For this review, take the finished solid that the model builds, in its own axes (mm). Round coordinates to 2 decimals unless told otherwise and drop trailing zeros. Loops run counter-clockwise (first coordinate to the right, second up) from the corner with the lowest first, then second, coordinate; pieces in that order, holes last. Notation, with made-up numbers: (42.25, 89) -> (47.25, 89) arc R8 ccw to (47.25, 95) -> close; hole circle Ø8 at (9, -16.5). An arc over 180 degrees is marked (long way). Use one line per item in the form item = value. Start each with the question number.
from build123d import *

# Parameters (mm, degrees)
F1_DEPTH = 20
F2_R     = 5
F4_DEPTH = 18


with BuildPart() as f1:
    # F0 (on Top) → F1 (new body)
    with BuildSketch(Plane.XY):
        Polygon((3.5849593993, 10.2129992476), (-4.6867319226, 9.7566301257), (-10.2129992476, 3.5849593993), (-9.7566301257, -4.6867319226), (-3.5849593993, -10.2129992476), (0, 0), (9.7566301257, 4.6867319226), align=None)
    extrude(amount=-F1_DEPTH)

    # F2
    f2_edges = [f1.edges().sort_by_distance(p)[0] for p in [
        (-3.584959, -10.212999, -10),
        (0, 0, -10),
        (-1.79248, -5.1065, 0),
        (-1.79248, -5.1065, -20),
        (9.75663, 4.686732, -10),
        (4.878315, 2.343366, 0),
        (4.878315, 2.343366, -20),
    ]]
    fillet(f2_edges, radius=F2_R)

    # F3 (on face) → F4 (cut)
    with BuildSketch(Plane.XY):
        with BuildLine():
            ThreePointArc((-5.4696709775, -0.4859568461), (-1.774196959, -0.43586708), (0.0592308539, 2.7731171302))
            ThreePointArc((0.0592308539, 2.7731171302), (-0.1609705435, 4.0348666123), (-0.7955405584, 5.1474407928))
            ThreePointArc((-0.7955405584, 5.1474407928), (-3.6017445612, 2.8495453067), (-5.4037427691, -0.2981374964))
            Line((-5.4037427691, -0.2981374964), (-5.4696709775, -0.4859568461))
        make_face()
        with BuildLine():
            ThreePointArc((-5.4037427691, -0.2981374964), (-3.6017445612, 2.8495453067), (-0.7955405584, 5.1474407928))
            ThreePointArc((-0.7955405584, 5.1474407928), (-6.5324842395, 5.1516817337), (-5.4696709775, -0.4859568461))
            Line((-5.4696709775, -0.4859568461), (-5.4037427691, -0.2981374964))
        make_face()
    extrude(amount=-F4_DEPTH, mode=Mode.SUBTRACT)


solid = f1.part
Item 1: For P1, Ø10, axis at y = -1.5, z = -6, coming from the +X side; P2, Ø2, axis at y = -1, z = -8, coming from the +X side; P3, Ø4, axis at x = 1, y = 1.5, coming from the +Z side; P4, Ø1, axis at x = 0, y = -3.5, coming from the +Z side, all flat-tipped, find the tip position at first contact; note any pin that passes through.
Item 2: Take a section at C-C on y = 8.5. Give the boundary of the cut face in (x, z).
Item 3: Wall thickness on line 1 (Z direction, x = -6, y = 4.75); line 2 (Y direction, x = -3, z = -13.75); line 3 (X direction, y = 0, z = -15): over which ranges is each line inside the solid? List them lowest first.
Item 4: Draft analysis for pull direction X (two halves, no side actions). For faces 1 (the cylindrical face through (-4.647, -6.356, -10.14)), 2 (the flat face through (-0.9, -2.56, -9.93)), 3 (the flat face through (-4, 3, -18)), 4 (the flat face through (-9.99, -0.49, -9.86)), state which applies: +X half, -X half, draft (parallel to the pull), parting line (faces both ways), or undercut.
Results:
q1.P1 = 5.2
q1.P2 = 0.57
q1.P3 = -0.44
q1.P4 = through
q2.outline = (-5.81, -20) -> (5.15, -20) -> (5.15, 0) -> (-5.81, 0) -> close
q3.line_1 = -20 to -18
q3.line_2 = -5.62 to -0.89, 6.44 to 9.85
q3.line_3 = -10.02 to -6.15, -1.18 to 0.57
q4.face_1 = parting line
q4.face_2 = +X half
q4.face_3 = undercut
q4.face_4 = -X half
